Geometry check sheet. Reference: the model listing, model coordinates, mm. Round coordinates to 2 decimals unless told otherwise and drop trailing zeros. Order: outer loops, then holes, each group sorted by start corner. A loop starts at its lowest first (then second) coordinate and runs counter-clockwise, first axis right, second up. Notation, with made-up numbers: (-24.75, -38) -> (2.25, -38) arc R31 cw to (2.25, -10) -> close; hole circle Ø7 at (40.25, 6.5). An arc over 180 degrees is marked (long way). Use a Markdown table: item, result. Add a question column.
Item 1: Sectioned sample at B-B, the plane z = 7.5. Record the cut outline in (x, y).
Item 2: Sectioned sample at A-A, the plane y = -11.5. Record the cut outline in (x, z).
Item 3: Material ranges on probe 1 along X at (y, z) = (9, 7.25); probe 2 along X at (y, z) = (7.5, 3.75); probe 3 along Y at (x, z) = (14, 22), recorded low to high. Write a range as [from, to].
Item 4: Mould release check, pull along X, two halves, no side actions. Record for faces 1 (the flat face through (-13.374, -2, 13)), 2 (the cylindrical face through (-8.21, -14.43, 13.27)), 3 (the flat face through (2, -6, 0)): pulls with the +X half, pulls with the -X half, needs draft (parallel to the pull), parting line crosses it, or undercut.
Item 5: Gauge pin test, flat ends, axial feed: pin 1 Ø1 at (x, z) = (-4.5, 15.5) entering from -Y; pin 2 Ø2 at (x, z) = (-8, 6.5) entering from +Y. Record the tip position at first contact, or that the pin passes through.
Item 6: Sectioned sample at D-D, the plane x = 1. Record the cut outline in (y, z), and give its area (3 significant figures).
Item 7: Sectioned sample at C-C, the plane y = -6. Record the cut outline in (x, z).
from build123d import *

# Parameters (mm, degrees)
F1_DEPTH = 26.92


with BuildPart() as f1:
    # F0 (on Top) → F1 (new body)
    with BuildSketch(Plane.XY):
        with BuildLine():
            ThreePointArc((-11.241594, 18.364918), (-12.292704, 19.320588), (-13.373895, 18.399088))
            Line((-13.373895, 18.399088), (-13.373895, -22.575411))
            Line((-13.373895, -22.575411), (18.626105, -23.408137))
            Line((18.626105, -23.408137), (18.626105, 18.379824))
            ThreePointArc((18.626105, 18.379824), (17.824413, 18.44657), (17.392959, 17.767591))
            Line((17.392959, 17.767591), (16.720654, -12.537674))
            ThreePointArc((16.720654, -12.537674), (14.131955, -15.124464), (11.545165, -12.535765))
            Line((11.545165, -12.535765), (11.277532, 18.364451))
            ThreePointArc((11.277532, 18.364451), (10.550878, 19.085636), (9.822628, 18.366063))
            Line((9.822628, 18.366063), (9.323563, -12.535565))
            ThreePointArc((9.323563, -12.535565), (6.76096, -15.09974), (4.196786, -12.537137))
            Line((4.196786, -12.537137), (3.699317, 18.3712))
            ThreePointArc((3.699317, 18.3712), (2.92693, 19.128157), (2.160752, 18.364918))
            Line((2.160752, 18.364918), (1.663561, -12.535565))
            ThreePointArc((1.663561, -12.535565), (-0.932977, -14.543026), (-3.529515, -12.535565))
            Line((-3.529515, -12.535565), (-3.79715, 18.364918))
            ThreePointArc((-3.79715, 18.364918), (-4.670126, 19.249776), (-5.581484, 18.404502))
            Line((-5.581484, 18.404502), (-5.8192, -12.535565))
            ThreePointArc((-5.8192, -12.535565), (-8.252189, -14.43033), (-10.685177, -12.535565))
            Line((-10.685177, -12.535565), (-11.241594, 18.364918))
        make_face()
    extrude(amount=F1_DEPTH)


solid = f1.part
Found:
| question | item | result |
|---|---|---|
| 1 | outline | (-13.37, -22.58) -> (18.63, -23.41) -> (18.63, 18.38) arc R0.78 ccw to (17.39, 17.77) -> (16.72, -12.54) arc R2.59 cw to (11.55, -12.54) -> (11.28, 18.36) arc R0.73 ccw to (9.82, 18.37) -> (9.32, -12.54) arc R2.56 cw to (4.2, -12.54) -> (3.7, 18.37) arc R0.77 ccw to (2.16, 18.36) -> (1.66, -12.54) arc R2.68 cw to (-3.53, -12.54) -> (-3.8, 18.36) arc R0.89 ccw to (-5.58, 18.4) -> (-5.82, -12.54) arc R2.51 cw to (-10.69, -12.54) -> (-11.24, 18.36) arc R1.07 ccw to (-13.37, 18.4) -> close |
| 2 | outline | (-13.37, 0) -> (-10.7, 0) -> (-10.7, 26.92) -> (-13.37, 26.92) -> close; (-5.81, 0) -> (-3.54, 0) -> (-3.54, 26.92) -> (-5.81, 26.92) -> close; (1.68, 0) -> (4.18, 0) -> (4.18, 26.92) -> (1.68, 26.92) -> close; (9.34, 0) -> (11.54, 0) -> (11.54, 26.92) -> (9.34, 26.92) -> close; (16.74, 0) -> (18.63, 0) -> (18.63, 26.92) -> (16.74, 26.92) -> close |
| 3 | probe 1 | x = [-13.37, -11.07], [-5.65, -3.72], [2.01, 3.85], [9.67, 11.36], [17.2, 18.63] |
| 3 | probe 2 | x = [-13.37, -11.05], [-5.67, -3.7], [1.99, 3.87], [9.65, 11.37], [17.17, 18.63] |
| 3 | probe 3 | y = [-23.29, -15.12] |
| 4 | face 1 | pulls with the -X half |
| 4 | face 2 | undercut |
| 4 | face 3 | needs draft |
| 5 | pin 1 | stops at y = -22.82 |
| 5 | pin 2 | stops at y = -14.1 |
| 6 | outline | (-22.95, 0) -> (-13.72, 0) -> (-13.72, 26.92) -> (-22.95, 26.92) -> close |
| 6 | area | 248 mm2 |
| 7 | outline | (-13.37, 0) -> (-10.8, 0) -> (-10.8, 26.92) -> (-13.37, 26.92) -> close; (-5.77, 0) -> (-3.59, 0) -> (-3.59, 26.92) -> (-5.77, 26.92) -> close; (1.77, 0) -> (4.09, 0) -> (4.09, 26.92) -> (1.77, 26.92) -> close; (9.43, 0) -> (11.49, 0) -> (11.49, 26.92) -> (9.43, 26.92) -> close; (16.87, 0) -> (18.63, 0) -> (18.63, 26.92) -> (16.87, 26.92) -> close |
